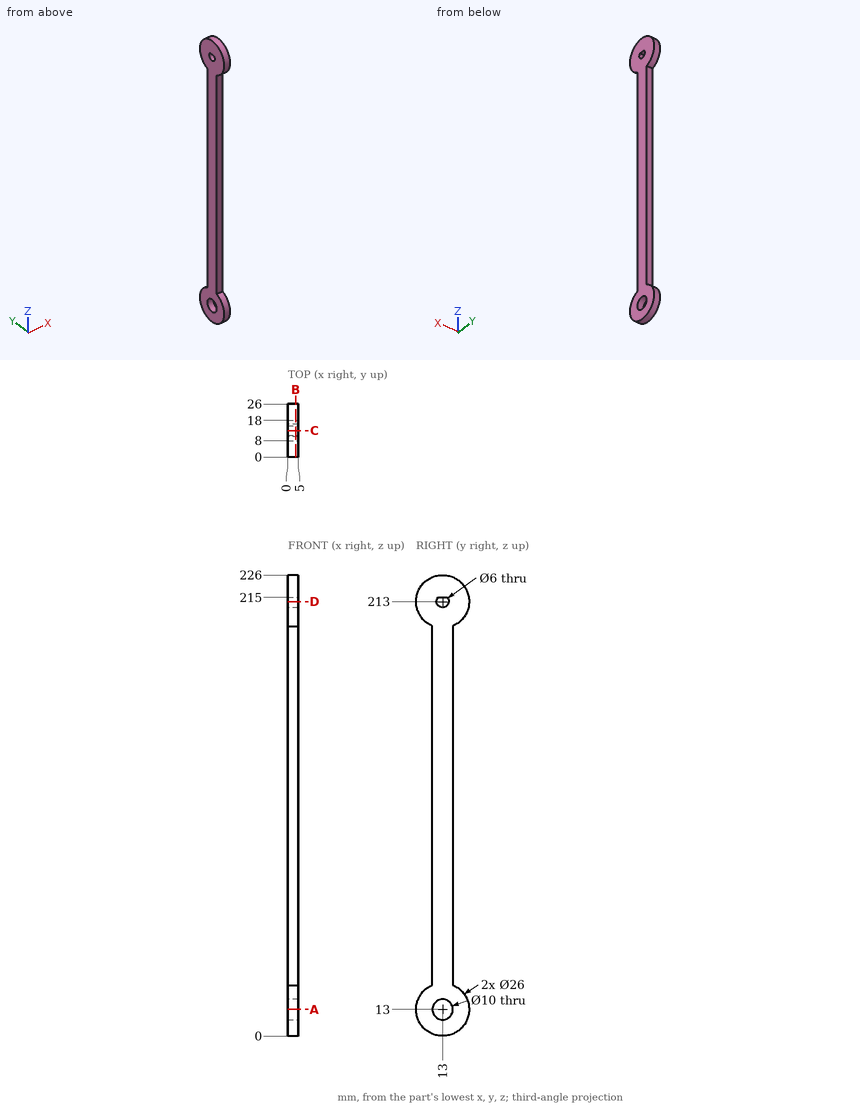
Could you check a few things on this drawing? It's one solid part, dimensions in mm from its lowest x, y, z. Coordinates: 2 decimals unless noted, no trailing zeros. Order: outer loops, then holes, each group sorted by start corner. A loop starts at its lowest first (then second) coordinate and runs counter-clockwise, first axis right, second up. Notation, with made-up numbers: (-34.5, -27) -> (15.5, -27) arc R7 ccw to (15.5, -15) -> close; hole circle Ø4 at (88, 44.5). An arc over 180 degrees is marked (long way). Answer in a Markdown table with one row per item.
(1) I want a section at C-C on y = 13. List the corners of the cut face in (x, z) for me, then the cut area to 4 significant figures.
Answer key:
| item | result |
|---|---|
| outline | (0, 0) -> (5, 0) -> (5, 8) -> (0, 8) -> close; (0, 18) -> (5, 18) -> (5, 210) -> (0, 210) -> close; (0, 215) -> (5, 215) -> (5, 226) -> (0, 226) -> close |
| area | 1,055 mm^2 |
(2) I want a section at A-A on z = 13. List the corners of the cut face in (x, y) for me, then the cut area to 3 significant figures.
Answer key:
| item | result |
|---|---|
| outline | (0, 0) -> (5, 0) -> (5, 8) -> (0, 8) -> close; (0, 18) -> (5, 18) -> (5, 26) -> (0, 26) -> close |
| area | 80.0 mm^2 |
(3) Please list where these lines run through material, in increasing order: probe 1 along Z at (x, y) = (4.5, 15.75); probe 2 along Z at (x, y) = (1.4, 10.5); probe 3 along Y at (x, z) = (2.55, 13).
Answer key:
| item | result |
|---|---|
| probe 1 | 0.29 to 8.82, 17.18 to 211.8, 214.2 to 225.71 |
| probe 2 | 0.24 to 8.67, 17.33 to 211.34, 214.66 to 225.76 |
| probe 3 | 0 to 8, 18 to 26 |
(4) I want a section at D-D on z = 213. List the corners of the cut face in (x, y) for me, then the cut area to 3 significant figures.
Answer key:
| item | result |
|---|---|
| outline | (0, 0) -> (5, 0) -> (5, 10) -> (0, 10) -> close; (0, 16) -> (5, 16) -> (5, 26) -> (0, 26) -> close |
| area | 100 mm^2 |
(5) I want a section at B-B on x = 3.75. List the corners of the cut face in (y, z) for me.
Answer key:
| item | result |
|---|---|
| outline | (8, 25) arc R13 ccw (long way) to (18, 25) -> (18, 201) arc R13 ccw (long way) to (8, 201) -> close; hole circle Ø10 at (13, 13); hole (10.76, 215) arc R3 ccw (long way) to (15.24, 215) -> close |
(6) Will these pins go through, and if not, where does the flat tip stop? pin 1 Ø2 at (x, z) = (1.5, 28) entering from +Y; pin 2 Ø1.5 at (x, z) = (2, 142.5) entering from -Y; pin 3 Ø1 at (x, y) = (2, 19.5) entering from +Z.
Answer key:
| item | result |
|---|---|
| pin 1 | y = 18 |
| pin 2 | y = 8 |
| pin 3 | z = 224.53 |
